Work out the finished part from the listing and answer in its coordinate system (mm). Coordinates: 2 decimals unless noted, no trailing zeros. Order: outer loops, then holes, each group sorted by start corner. A loop starts at its lowest first (then second) coordinate and runs counter-clockwise, first axis right, second up. Notation, with made-up numbers: M 84.25,42 L 138.25,42 A13 ccw 138.25,48 Z; hole C -1,51 d7. An arc over 180 degrees is marked long. Use a Markdown table: item, result.
from build123d import *

# Parameters (mm, degrees)
F2_R     = 2.5
F3_DEPTH = 25


with BuildPart() as f1:
    # F0 (on Front) → F1 (revolve)
    with BuildSketch(Plane.XZ):
        with BuildLine():
            Line((195, 0), (214.8, 0))
            Line((214.8, 0), (214.8, 15))
            Line((214.8, 15), (170, 15))
            Line((170, 15), (170, 0))
            Line((170, 0), (190.003342, 0))
            ThreePointArc((190.003342, 0), (192.501671, 2.591396), (195, 0))
        make_face()
    revolve(axis=Axis((0, 0, 19.496838), (0, 0, 1)))

    # F2 (on face) → F3 (cut)
    with BuildSketch(Plane.XY.offset(15)):
        with Locations((205.8, 0)):
            Circle(F2_R)
        with Locations((0, 205.8)):
            Circle(F2_R)
        with Locations((-205.8, 0)):
            Circle(F2_R)
        with Locations((0, -205.8)):
            Circle(F2_R)
    extrude(amount=-F3_DEPTH, mode=Mode.SUBTRACT)


solid = f1.part
(1) A cutting plane is placed at A-A (z = 8). Determine the outline of the cut face in (x, y).
Conclusion:
| item | result |
|---|---|
| outline | C 0,0 d429.6; hole C -205.8,0 d5; hole C 0,0 d340; hole C 0,-205.8 d5; hole C 0,205.8 d5; hole C 205.8,0 d5 |
(2) Straight lines are drawn through the part: L1, parallel to Y at x = 0, z = 4.5; L2, parallel to X at y = -62.5, z = 1; L3, parallel to X at y = 75.5, z = 1.25. For each, find the intervals that lie inside material, in ascending order.
Conclusion:
| item | result |
|---|---|
| L1 | -214.8 to -208.3, -203.3 to -170, 170 to 203.3, 208.3 to 214.8 |
| L2 | -205.51 to -184.53, -179.61 to -158.09, 158.09 to 179.61, 184.53 to 205.51 |
| L3 | -201.09 to -179.48, -174.67 to -152.31, 152.31 to 174.67, 179.48 to 201.09 |
(3) Determine the mould class of faces 1 (the cylindrical face through (-158.32, 145.17, 7.6)), 2 (the flat face through (-190, -47, 0)), 3 (the cylindrical face through (-134.91, -103.44, 7.4)) for opening direction Y: pulls with the +Y half, pulls with the -Y half, needs draft (parallel to the pull), parting line crosses it, or undercut.
Conclusion:
| item | result |
|---|---|
| face 1 | parting line crosses it |
| face 2 | needs draft |
| face 3 | undercut |
(4) Given P1, Ø4, axis at x = 205.8, y = 0, coming from the -Z side; P2, Ø8, axis at x = 22, z = 7, coming from the -Y side; P3, Ø1.5, axis at x = -50.5, z = 9, coming from the -Y side, each flat-ended and moving along its own axis, determine where each tip first touches the part or whether it passes through.
Conclusion:
| item | result |
|---|---|
| P1 | through |
| P2 | y = -214.04 |
| P3 | y = -208.96 |
